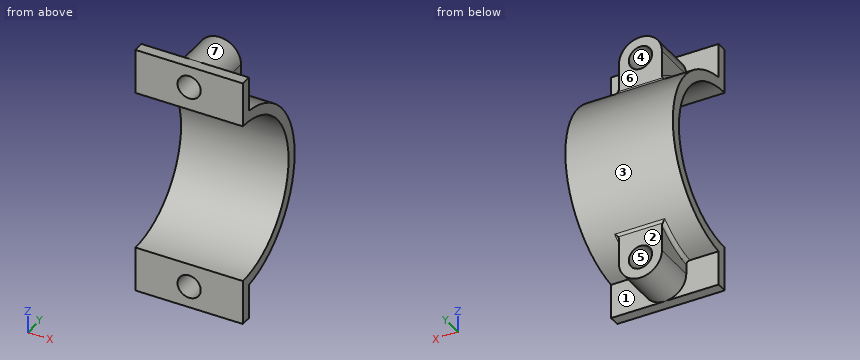
from build123d import *

# Parameters (mm, degrees)
BOSS_EXTRUDE1_DEPTH = 15
BOSS_EXTRUDE2_REACH = 42.927
SKETCH3_R           = 3.25
CUT_EXTRUDE1_DEPTH  = 41.926763859
FILLET1_R           = 1


with BuildPart() as part:
    # Sketch1 → Boss-Extrude1 (new, symmetric)
    with BuildSketch(Plane(origin=(0, 0, 0), x_dir=(0, 0, -1), z_dir=(1, 0, 0))):
        with BuildLine():
            Line((-22.5, 0), (-35, 0))
            Line((-35, 0), (-35, 3))
            Line((-35, 3), (-25.322914524, 3))
            ThreePointArc((-25.322914524, 3), (0, 25.5), (25.322914524, 3))
            Line((25.322914524, 3), (35, 3))
            Line((35, 3), (35, 0))
            Line((35, 0), (22.5, 0))
            ThreePointArc((22.5, 0), (0, 22.5), (-22.5, 0))
        make_face()
    extrude(amount=BOSS_EXTRUDE1_DEPTH, both=True)

    # Sketch2 → Boss-Extrude2 (add, up to next)
    with BuildSketch(Plane(origin=(0, 15, 0), x_dir=(1, 0, 0), z_dir=(0, 1, 0)), mode=Mode.PRIVATE) as boss_extrude2_sk1:
        with BuildLine():
            Line((-6, -29), (-6, -19))
            Line((-6, -19), (6, -19))
            Line((6, -19), (6, -29))
            ThreePointArc((6, -29), (0, -35), (-6, -29))
        make_face()
    boss_extrude2_tool1 = extrude(boss_extrude2_sk1.sketch, amount=-BOSS_EXTRUDE2_REACH, mode=Mode.PRIVATE) - part.part
    boss_extrude2 = boss_extrude2_tool1.solids().sort_by_distance((0, 15, 26.417143))[0]
    add(boss_extrude2)

    # Sketch3 → Cut-Extrude1 (cut, through all)
    with BuildSketch(Plane(origin=(0, 15, 0), x_dir=(1, 0, 0), z_dir=(0, 1, 0))):
        with Locations(Location((0, -29, 0), (0, 0, 270))):
            Circle(SKETCH3_R)
    cut_extrude1 = extrude(amount=-CUT_EXTRUDE1_DEPTH, mode=Mode.SUBTRACT)

    # Mirror1: Boss-Extrude2, Cut-Extrude1 across plane
    add(boss_extrude2.mirror(Plane.XY))
    add(cut_extrude1.mirror(Plane.XY), mode=Mode.SUBTRACT)

    # Fillet1
    fillet1_edges = [part.edges().sort_by_distance(p)[0] for p in [
        (-6, 9.301914405, 23.742880794),
        (6, 9.301914405, 23.742880794),
        (0, 15, 20.621590627),
        (-6, 9.301914405, -23.742880794),
        (6, 9.301914405, -23.742880794),
        (0, 15, -20.621590627),
    ]]
    fillet(fillet1_edges, radius=FILLET1_R)


solid = part.part
Input: part model. Units: mm. Frame: model coordinates. Face numbers are marked on the shaded views. A direction names the side the tool comes from. Coordinates: 2 decimals unless noted, no trailing zeros. Loops run counter-clockwise (first coordinate to the right, second up) from the corner with the lowest first, then second, coordinate; pieces in that order, holes last.
(1) Pull-direction query (X, two-part tool) for the marked faces 4, 5, 6 and 7; classes: released by +X, released by -X, zero draft, split by the parting line, or undercut.
(2) Section C-C on x = -11. Return the cut outline in (y, z).
(3) Set-up query: the marked faces 1, 2 and 3. Return all of +Z, -Z, +X, -X, +Y, -Y with unobstructed straight access to the full face (end or side cutting, diameter ignored); none if empty.
(4) Material intervals for probe 1 along X at (y, z) = (8.5, -29); probe 2 along Y at (x, z) = (6, 31); probe 3 along X at (y, z) = (7, 31), sorted ascending.
(5) Section B-B on y = 16.5. Return the cut outline in (x, z), then the cut area to 3 significant figures.
(6) Section D-D on y = 13.25. Count the separate pieces of the cut face and the enclosed holes in it, then the cut area to 3 significant figures.
(7) Section A-A on z = -28. Return the cut outline in (x, y).
(8) First-contact query: pin 1 Ø6 at (x, z) = (0.5, 27) entering from +Y; pin 2 Ø2 at (x, y) = (2, 13.5) entering from +Z; pin 3 Ø6 at (x, y) = (-8, 7.5) entering from -Z. Flat tips, straight axial feed; report the tip coordinate or a pass-through.
Data:
1. face 4: undercut
1. face 5: undercut
1. face 6: zero draft
1. face 7: split by the parting line
2. outline: (0, -35) - (3, -35) - (3, -25.32) arc R25.5 ccw to (3, 25.32) - (3, 35) - (0, 35) - (0, 22.5) arc R22.5 cw to (0, -22.5) - close
3. face 1: -Z, +X, +Y
3. face 2: -Z, +X, -X, +Y
3. face 3: +Y
4. probe 1: x = -6 to -3.25, 3.25 to 6
4. probe 2: y = 0 to 3
4. probe 3: x = -5.66 to -2.56, 2.56 to 5.66
5. outline: (-15, -19.44) - (15, -19.44) - (15, -15.3) - (-15, -15.3) - close; (-15, 15.3) - (15, 15.3) - (15, 19.44) - (-15, 19.44) - close
5. area: 249 mm2
6. separate pieces: 2
6. enclosed holes: 2
6. area: 437 mm2
7. outline: (-15, 0) - (-3.09, 0) - (-3.09, 15) - (-6, 15) - (-6, 3) - (-15, 3) - close; (3.09, 0) - (15, 0) - (15, 3) - (6, 3) - (6, 15) - (3.09, 15) - close
8. pin 1: stops at y = 15
8. pin 2: stops at z = 34.92
8. pin 3: stops at z = -32.32
